Input: part model. Units: mm. Frame: model coordinates. A direction names the side the tool comes from. Give positions to 0.01 mm unless a question says otherwise; leave off trailing zeros. Loops run counter-clockwise (first coordinate to the right, second up) from the corner with the lowest first, then second, coordinate; pieces in that order, holes last. Notation, with made-up numbers: (33, 30) -> (67, 30) arc R15 cw to (67, 55) -> close; hole circle Ø10 at (30.5, 6). An arc over 180 degrees is marked (long way). One line per question, with ' | ' between items.
from build123d import *

# Parameters (mm, degrees)
SKETCH_1_W          = 30
SKETCH_1_H          = 50
SKETCH_1_R          = 3.5
SKETCH_1_R_2        = 4.25
EXTRUDE_1_DEPTH     = 22
SKETCH_2_R          = 12.9
CUT_EXTRUDE_1_DEPTH = 5
SKETCH_3_R          = 6
CUT_EXTRUDE_2_DEPTH = 3.5
SKETCH_4_R          = 7
CUT_EXTRUDE_3_DEPTH = 5


with BuildPart() as part:
    # 草图1 → 凸台-拉伸1 (new body)
    with BuildSketch(Plane(origin=(0, 0, 0), x_dir=(1, 0, 0), z_dir=(0, 1, 0))):
        Rectangle(SKETCH_1_W, SKETCH_1_H)
        with Locations((0, -9.125)):
            Circle(SKETCH_1_R, mode=Mode.SUBTRACT)
        with Locations((0, 15.25)):
            Circle(SKETCH_1_R_2, mode=Mode.SUBTRACT)
    extrude(amount=EXTRUDE_1_DEPTH)

    # 草图2 → 切除-拉伸1 (cut)
    with BuildSketch(Plane(origin=(0, 22, 0), x_dir=(1, 0, 0), z_dir=(0, 1, 0))):
        with Locations((0, -9.125)):
            Circle(SKETCH_2_R)
    extrude(amount=-CUT_EXTRUDE_1_DEPTH, mode=Mode.SUBTRACT)

    # 草图3 → 切除-拉伸2 (cut)
    with BuildSketch(Plane.XZ):
        with Locations((0, 9.125)):
            Circle(SKETCH_3_R)
    extrude(amount=-CUT_EXTRUDE_2_DEPTH, mode=Mode.SUBTRACT)

    # 草图4 → 切除-拉伸3 (cut)
    with BuildSketch(Plane(origin=(0, 22, 0), x_dir=(1, 0, 0), z_dir=(0, 1, 0))):
        with Locations((0, 15.25)):
            Circle(SKETCH_4_R)
    extrude(amount=-CUT_EXTRUDE_3_DEPTH, mode=Mode.SUBTRACT)


solid = part.part
1. Section query D-D (x = -10.5). Output: boundary loops of the cut face in (y, z), then the cut area to 3 significant figures.
Determined:
outline: (0, -25) -> (22, -25) -> (22, 1.63) -> (17, 1.63) -> (17, 16.62) -> (22, 16.62) -> (22, 25) -> (0, 25) -> close | area: 1,030 mm2
2. Section query B-B (x = 0). Output: boundary loops of the cut face in (y, z) (3 decimals).
Determined:
outline: (0, -25) -> (22, -25) -> (22, -22.25) -> (17, -22.25) -> (17, -19.5) -> (0, -19.5) -> close; (0, -11) -> (17, -11) -> (17, -8.25) -> (22, -8.25) -> (22, -3.775) -> (17, -3.775) -> (17, 5.625) -> (3.5, 5.625) -> (3.5, 3.125) -> (0, 3.125) -> close; (0, 15.125) -> (3.5, 15.125) -> (3.5, 12.625) -> (17, 12.625) -> (17, 22.025) -> (22, 22.025) -> (22, 25) -> (0, 25) -> close
3. Section query C-C (y = 8.25). Output: boundary loops of the cut face in (x, z) (3 decimals).
Determined:
outline: (-15, -25) -> (15, -25) -> (15, 25) -> (-15, 25) -> close; hole circle Ø8.5 at (0, -15.25); hole circle Ø7 at (0, 9.125)
4. Ray query, line 1 along Z through (x, y) = (0, 12.25) (3 decimals); line 2 along Z through (x, y) = (0, 1.9) (3 decimals); line 3 along X through (y, z) = (18.85, -15.25). Return the intervals inside material, ascending. Write a range as from..to.
Determined:
line 1: z = -25..-19.5, -11..5.625, 12.625..25 | line 2: z = -25..-19.5, -11..3.125, 15.125..25 | line 3: x = -15..-7, 7..15
5. Reachability of faces 5 (the cylindrical face through (12.304, 19.535, 5.25)), 6 (the cylindrical face through (-0.76, 10.16, 12.54)), 7 (the cylindrical face through (-1.301, 1.726, 3.268)) from +Z, -Z, +X, -X, +Y, -Y: full face, straight path, thin tool, end or side. Return the list, or none.
Determined:
face 5: +Y | face 6: +Y, -Y | face 7: -Y
6. Pin query (flat end, axial travel): P1, Ø3, axis at x = -10, z = 12.5, coming from the +Y side; P2, Ø7, axis at x = 0, z = -15.25, coming from the -Y side. Return the tip coordinate at first contact, or that it passes through.
Determined:
P1: stops at y = 17 | P2: passes through
7. Pull-direction query (X, two-part tool) for faces 1 (the flat face through (3, 17, -12)), 2 (the flat face through (0, 0, 0)), 3 (the flat face through (3, 3.5, 7)), 4 (the flat face through (-15, 11, 0)); classes: pulls with the +X half, pulls with the -X half, needs draft (parallel to the pull), parting line crosses it, or undercut.
Determined:
face 1: undercut | face 2: needs draft | face 3: undercut | face 4: pulls with the -X half
8. Section query A-A (z = -15.25). Output: boundary loops of the cut face in (x, y), then the cut area to 4 significant figures.
Determined:
outline: (-15, 0) -> (-4.25, 0) -> (-4.25, 17) -> (-7, 17) -> (-7, 22) -> (-15, 22) -> close; (4.25, 0) -> (15, 0) -> (15, 22) -> (7, 22) -> (7, 17) -> (4.25, 17) -> close | area: 445.5 mm2
